```python
from build123d import *

# Parameters (mm, degrees)
BOSS_EXTRUDE1_DEPTH            = 3
SKETCH3_R                      = 4
CUT_EXTRUDE1_DEPTH             = 3
CBORE_FOR_M2_SHCS1_D           = 2.4
CBORE_FOR_M2_SHCS1_DEPTH       = 3
CBORE_FOR_M2_SHCS1_CBORE_D     = 4.4
CBORE_FOR_M2_SHCS1_CBORE_DEPTH = 2
CBORE_FOR_M2_SHCS1_TIP         = 0.721032743
CUT_EXTRUDE2_DEPTH             = 3
SKETCH7_W                      = 6
SKETCH7_H                      = 10
CUT_EXTRUDE3_DEPTH             = 3
CUT_EXTRUDE4_DEPTH             = 3
CBORE_FOR_M2_SHCS2_D           = 2.4
CBORE_FOR_M2_SHCS2_DEPTH       = 3
CBORE_FOR_M2_SHCS2_CBORE_D     = 4.4
CBORE_FOR_M2_SHCS2_CBORE_DEPTH = 2
CBORE_FOR_M2_SHCS2_TIP         = 0.721032743
SALIENTE_EXTRUIR2_DEPTH        = 3
CORTAR_EXTRUIR2_DEPTH          = 25
CORTAR_EXTRUIR3_DEPTH          = 8
CORTAR_EXTRUIR3_DEPTH_BACK     = 1
SALIENTE_EXTRUIR3_DEPTH        = 3
CORTAR_EXTRUIR4_DEPTH          = 32
CORTAR_EXTRUIR4_DEPTH_BACK     = 3
CORTAR_EXTRUIR5_DEPTH          = 33
CORTAR_EXTRUIR5_DEPTH_BACK     = 16
CORTAR_EXTRUIR6_DEPTH          = 36
CORTAR_EXTRUIR6_DEPTH_BACK     = 57
CROQUIS10_W                    = 8
CROQUIS10_H                    = 20.24327749
CROQUIS11_W                    = 22.516217108
CROQUIS11_H                    = 6.585791746
SALIENTE_EXTRUIR4_DEPTH        = 3
CORTAR_EXTRUIR7_DEPTH          = 12
CORTAR_EXTRUIR7_DEPTH_BACK     = 26
CORTAR_EXTRUIR8_DEPTH          = 37
CORTAR_EXTRUIR8_DEPTH_BACK     = 23
CORTAR_EXTRUIR10_DEPTH         = 10
CORTAR_EXTRUIR10_DEPTH_BACK    = 13
CROQUIS14_W                    = 22.056135014
CROQUIS14_H                    = 3.895510455
CORTAR_EXTRUIR11_DEPTH         = 15
CORTAR_EXTRUIR11_DEPTH_BACK    = 12
CROQUIS15_W                    = 4.816352665
CROQUIS15_H                    = 5.664480242
CORTAR_EXTRUIR12_DEPTH         = 33
CORTAR_EXTRUIR12_DEPTH_BACK    = 21
CORTAR_EXTRUIR18_DEPTH         = 52
CORTAR_EXTRUIR18_DEPTH_BACK    = 75
CORTAR_EXTRUIR19_DEPTH         = 24
CORTAR_EXTRUIR19_DEPTH_BACK    = 67
CORTAR_EXTRUIR20_DEPTH         = 39
CORTAR_EXTRUIR20_DEPTH_BACK    = 62
SALIENTE_EXTRUIR7_DEPTH        = 3
SALIENTE_EXTRUIR9_DEPTH        = 3
SALIENTE_EXTRUIR10_DEPTH       = 3


with BuildPart() as part:
    # Sketch2 → Boss-Extrude1 (new body)
    with BuildSketch(Plane.XY):
        Polygon((-5.811176978, -98.599598559), (-3.564526654, -100.58433119), (7.435473346, -100.58433119), (9.68212367, -98.599598559), (21.318847535, -4.961831578), (21.935473346, 5), (21.935473346, 45), (21.193771081, 54.944681764), (15.17717561, 95.055318236), (9.435473346, 100), (-5.564526654, 100), (-11.306228919, 95.055318236), (-17.32282439, 54.944681764), (-18.064526654, 45), (-18.064526654, 5), (-17.447900844, -4.961831578), align=None)
    extrude(amount=BOSS_EXTRUDE1_DEPTH)

    # Sketch3 → Cut-Extrude1 (cut)
    with BuildSketch(Plane.XY.offset(3)):
        with Locations((1.935473346, 25)):
            Circle(SKETCH3_R)
    extrude(amount=-CUT_EXTRUDE1_DEPTH, mode=Mode.SUBTRACT)

    # CBORE for M2 SHCS1
    with Locations(Plane.XY.offset(3)):
        with Locations((1.935473346, 33), (9.935473346, 25), (1.935473346, 17), (-6.064526654, 25)):
            CounterBoreHole(CBORE_FOR_M2_SHCS1_D / 2, CBORE_FOR_M2_SHCS1_CBORE_D / 2, CBORE_FOR_M2_SHCS1_CBORE_DEPTH, depth=CBORE_FOR_M2_SHCS1_DEPTH)
            with Locations((0, 0, -(CBORE_FOR_M2_SHCS1_DEPTH + CBORE_FOR_M2_SHCS1_TIP / 2))):  # 118° drill point
                Cone(0, CBORE_FOR_M2_SHCS1_D / 2, CBORE_FOR_M2_SHCS1_TIP, mode=Mode.SUBTRACT)

    # Sketch6 → Cut-Extrude2 (cut)
    with BuildSketch(Plane.XY.offset(3)):
        Polygon((-10.32282439, 54.944681764), (-2.592495206, 54.944681764), (-0.592495206, 56.944681764), (-0.592495206, 77.986977382), (-2.570367912, 80.283658288), (-6.413140682, 80.860074204), (-8.687694294, 79.178882404), (-12.026143484, 56.92255447), align=None)
        Polygon((15.841153071, 56.92255447), (12.502703881, 79.178882404), (10.22815027, 80.860074204), (6.385377499, 80.283658288), (4.407504794, 77.986977382), (4.407504794, 56.944681764), (6.407504794, 54.944681764), (14.137833977, 54.944681764), align=None)
        Polygon((-4.417484259, 94.313615971), (8.232493846, 94.313615971), (10.529174752, 92.335743265), (11.167639805, 88.07930958), (9.486448005, 85.804755968), (1.907504794, 84.667914487), (-5.671438417, 85.804755968), (-7.352630217, 88.07930958), (-6.714165164, 92.335743265), align=None)
    extrude(amount=-CUT_EXTRUDE2_DEPTH, mode=Mode.SUBTRACT)

    # Sketch7 → Cut-Extrude3 (cut)
    with BuildSketch(Plane.XY.offset(3)):
        with Locations((1.935473346, -85.58433119)):
            Rectangle(SKETCH7_W, SKETCH7_H)
    extrude(amount=-CUT_EXTRUDE3_DEPTH, mode=Mode.SUBTRACT)

    # Sketch8 → Cut-Extrude4 (cut)
    with BuildSketch(Plane.XY.offset(3)):
        Polygon((-8.447900844, -4.961831578), (12.318847535, -4.961831578), (1.935473346, -24.483157151), align=None)
        Polygon((15.880690917, -8.470858754), (8.202586605, -69.961831578), (4.435473346, -69.961831578), (4.435473346, -29.183297302), align=None)
        Polygon((-12.009744226, -8.470858754), (-4.331639914, -69.961831578), (-0.564526654, -69.961831578), (-0.564526654, -29.183297302), align=None)
    extrude(amount=-CUT_EXTRUDE4_DEPTH, mode=Mode.SUBTRACT)

    # CBORE for M2 SHCS2
    with Locations(Plane.XY.offset(3)):
        with Locations((-3.715014103, -74.923663156), (7.581217459, -74.961831578), (-11.190875883, -5.696432584), (15.095204577, -5.939721308), (1.907504794, 81.167914487)):
            CounterBoreHole(CBORE_FOR_M2_SHCS2_D / 2, CBORE_FOR_M2_SHCS2_CBORE_D / 2, CBORE_FOR_M2_SHCS2_CBORE_DEPTH, depth=CBORE_FOR_M2_SHCS2_DEPTH)
            with Locations((0, 0, -(CBORE_FOR_M2_SHCS2_DEPTH + CBORE_FOR_M2_SHCS2_TIP / 2))):  # 118° drill point
                Cone(0, CBORE_FOR_M2_SHCS2_D / 2, CBORE_FOR_M2_SHCS2_TIP, mode=Mode.SUBTRACT)

    # Croquis2 → Saliente-Extruir2 (add)
    with BuildSketch(Plane.XY):
        Polygon((18.794620774, 54.944681764), (-14.944396603, 54.944681764), (-7.478946257, 96.267482636), (12.143583194, 96.267482636), align=None)
    extrude(amount=SALIENTE_EXTRUIR2_DEPTH)

    # Croquis3 → Cortar-Extruir2 (cut)
    with BuildSketch(Plane.XY):
        Polygon((3.935473346, 75), (15.193771081, 54.944681764), (9.17717561, 95.055318236), (3.935473346, 95.055318236), align=None)
        Polygon((-5.306228919, 95.055318236), (-11.32282439, 54.944681764), (-0.064526654, 75), (-0.064526654, 95.055318236), align=None)
        Polygon((1.935473346, 67.392726007), (10.193771081, 54.944681764), (-6.32282439, 54.944681764), align=None)
    extrude(amount=CORTAR_EXTRUIR2_DEPTH, mode=Mode.SUBTRACT)

    # Croquis4 → Cortar-Extruir3 (cut, two sides: drawn at the far end of the back side and taken through both)
    with BuildSketch(Plane.XY.offset(-CORTAR_EXTRUIR3_DEPTH_BACK)):
        Polygon((-16.681169013, 74.945942972), (0, 74.945942972), (20.337076697, 74.945942972), (20.337076697, 106.026068233), (-16.681169013, 106.026068233), align=None)
    extrude(amount=CORTAR_EXTRUIR3_DEPTH + CORTAR_EXTRUIR3_DEPTH_BACK, mode=Mode.SUBTRACT)

    # Croquis5 → Saliente-Extruir3 (add)
    with BuildSketch(Plane.XY):
        Polygon((-14.322635208, 74.945942972), (18.1935819, 74.945942972), (18.1935819, 53.950721804), (-16.161111671, 53.950721804), align=None)
    extrude(amount=SALIENTE_EXTRUIR3_DEPTH)

    # Croquis8 → Cortar-Extruir4 (cut, two sides: drawn at the far end of the back side and taken through both)
    with BuildSketch(Plane.XY.offset(-CORTAR_EXTRUIR4_DEPTH_BACK)):
        Polygon((-14.322635208, 74.945942972), (-15.372635208, 67.945942972), (-9.322635208, 74.945942972), align=None)
        Polygon((18.1935819, 74.945942972), (13.1935819, 74.945942972), (19.2435819, 67.945942972), align=None)
    extrude(amount=CORTAR_EXTRUIR4_DEPTH + CORTAR_EXTRUIR4_DEPTH_BACK, mode=Mode.SUBTRACT)

    # Croquis9 → Cortar-Extruir5 (cut, two sides: drawn at the far end of the back side and taken through both)
    with BuildSketch(Plane.XY.offset(-CORTAR_EXTRUIR5_DEPTH_BACK)):
        Polygon((-9.322635208, 67.945942972), (-9.322635208, 70.912384295), (13.1935819, 70.912384295), (13.1935819, 67.945942972), (13.1935819, 64.326592549), (-9.322635208, 64.326592549), align=None)
    extrude(amount=CORTAR_EXTRUIR5_DEPTH + CORTAR_EXTRUIR5_DEPTH_BACK, mode=Mode.SUBTRACT)

    # Croquis10 → Cortar-Extruir6 (cut, two sides: drawn at the far end of the back side and taken through both)
    with BuildSketch(Plane.XY.offset(-CORTAR_EXTRUIR6_DEPTH_BACK)):
        with Locations((-5.322635208, 49.537038019)):
            Rectangle(CROQUIS10_W, CROQUIS10_H)
        with Locations((9.1935819, 49.537038019)):
            Rectangle(CROQUIS10_W, CROQUIS10_H)
    extrude(amount=CORTAR_EXTRUIR6_DEPTH + CORTAR_EXTRUIR6_DEPTH_BACK, mode=Mode.SUBTRACT)

    # Croquis11 → Saliente-Extruir4 (add)
    with BuildSketch(Plane.XY):
        with Locations((1.935473346, 67.619488422)):
            Rectangle(CROQUIS11_W, CROQUIS11_H)
    extrude(amount=SALIENTE_EXTRUIR4_DEPTH)

    # Croquis12 → Cortar-Extruir7 (cut, two sides: drawn at the far end of the back side and taken through both)
    with BuildSketch(Plane.XY.offset(-CORTAR_EXTRUIR7_DEPTH_BACK)):
        Polygon((-15.372635208, 67.945942972), (-9.322635208, 74.945942972), (-5.822635208, 74.945942972), (-17.32282439, 54.944681764), align=None)
    extrude(amount=CORTAR_EXTRUIR7_DEPTH + CORTAR_EXTRUIR7_DEPTH_BACK, mode=Mode.SUBTRACT)

    # Croquis13 → Cortar-Extruir8 (cut, two sides: drawn at the far end of the back side and taken through both)
    with BuildSketch(Plane.XY.offset(-CORTAR_EXTRUIR8_DEPTH_BACK)):
        Polygon((13.1935819, 74.945942972), (9.6935819, 74.945942972), (21.193771081, 54.944681764), (19.2435819, 67.945942972), align=None)
    extrude(amount=CORTAR_EXTRUIR8_DEPTH + CORTAR_EXTRUIR8_DEPTH_BACK, mode=Mode.SUBTRACT)

    # Croquis14 → Cortar-Extruir10 (cut, two sides: drawn at the far end of the back side and taken through both)
    with BuildSketch(Plane.XY.offset(-CORTAR_EXTRUIR10_DEPTH_BACK)):
        with Locations((5.205432299, 72.998187745)):
            Rectangle(CROQUIS14_W, CROQUIS14_H)
    extrude(amount=CORTAR_EXTRUIR10_DEPTH + CORTAR_EXTRUIR10_DEPTH_BACK, mode=Mode.SUBTRACT)

    # Croquis15 → Cortar-Extruir11 (cut, two sides: drawn at the far end of the back side and taken through both)
    with BuildSketch(Plane.XY.offset(-CORTAR_EXTRUIR11_DEPTH_BACK)):
        with Locations((-8.230811541, 73.882672638)):
            Rectangle(CROQUIS15_W, CROQUIS15_H)
    extrude(amount=CORTAR_EXTRUIR11_DEPTH + CORTAR_EXTRUIR11_DEPTH_BACK, mode=Mode.SUBTRACT)

    # Croquis16 → Cortar-Extruir12 (cut, two sides: drawn at the far end of the back side and taken through both)
    with BuildSketch(Plane.XY.offset(-CORTAR_EXTRUIR12_DEPTH_BACK)):
        Polygon((-8.062449324, 71.050432517), (-7.062449324, 71.050432517), (-17.32282439, 54.944681764), align=None)
        Polygon((11.933396016, 71.050432517), (10.933396016, 71.050432517), (21.193771081, 54.944681764), align=None)
    extrude(amount=CORTAR_EXTRUIR12_DEPTH + CORTAR_EXTRUIR12_DEPTH_BACK, mode=Mode.SUBTRACT)

    # Croquis18 → Cortar-Extruir18 (cut, two sides: drawn at the far end of the back side and taken through both)
    with BuildSketch(Plane.XY.offset(-CORTAR_EXTRUIR18_DEPTH_BACK)):
        Polygon((-7.062449324, 71.050432517), (-5.062449324, 71.050432517), (-7.826924714, 69.850432517), align=None)
        Polygon((10.933396016, 71.050432517), (8.933396016, 71.050432517), (11.697871405, 69.850432517), align=None)
    extrude(amount=CORTAR_EXTRUIR18_DEPTH + CORTAR_EXTRUIR18_DEPTH_BACK, mode=Mode.SUBTRACT)

    # Croquis20 → Cortar-Extruir19 (cut, two sides: drawn at the far end of the back side and taken through both)
    with BuildSketch(Plane.XY.offset(-CORTAR_EXTRUIR19_DEPTH_BACK)):
        Polygon((21.193771081, 54.944681764), (20.226639816, 56.462791483), (21.564622213, 49.972340882), align=None)
        Polygon((-17.32282439, 54.944681764), (-16.355693125, 56.462791483), (-17.693675522, 49.972340882), align=None)
    extrude(amount=CORTAR_EXTRUIR19_DEPTH + CORTAR_EXTRUIR19_DEPTH_BACK, mode=Mode.SUBTRACT)

    # Croquis21 → Cortar-Extruir20 (cut, two sides: drawn at the far end of the back side and taken through both)
    with BuildSketch(Plane.XY.offset(-CORTAR_EXTRUIR20_DEPTH_BACK)):
        Polygon((-9.322635208, 39.415399274), (-12.822635208, 39.415399274), (-9.322635208, 59.658676764), align=None)
        Polygon((13.1935819, 39.415399274), (16.6935819, 39.415399274), (13.1935819, 59.658676764), align=None)
    extrude(amount=CORTAR_EXTRUIR20_DEPTH + CORTAR_EXTRUIR20_DEPTH_BACK, mode=Mode.SUBTRACT)

    # Croquis23 → Saliente-Extruir7 (add)
    with BuildSketch(Plane.XY):
        Polygon((-9.322635208, 59.658676764), (-9.581980564, 58.158676764), (-7.822635208, 59.658676764), align=None)
        Polygon((13.1935819, 59.658676764), (11.6935819, 59.658676764), (13.452927256, 58.158676764), align=None)
    extrude(amount=SALIENTE_EXTRUIR7_DEPTH)

    # Croquis24 → Saliente-Extruir9 (add)
    with BuildSketch(Plane.XY):
        Polygon((-12.822635208, 39.415399274), (-11.022635208, 39.415399274), (-12.476841401, 41.415399274), align=None)
        Polygon((-1.322635208, 39.415399274), (-1.322635208, 40.415399274), (-2.322635208, 39.415399274), align=None)
        Polygon((5.1935819, 39.415399274), (6.1935819, 39.415399274), (5.1935819, 40.415399274), align=None)
        Polygon((14.8935819, 39.415399274), (16.347788092, 41.415399274), (16.6935819, 39.415399274), align=None)
    extrude(amount=SALIENTE_EXTRUIR9_DEPTH)

    # Croquis25 → Saliente-Extruir10 (add)
    with BuildSketch(Plane.XY):
        Polygon((5.1935819, 59.658676764), (5.1935819, 58.658676764), (7.1935819, 59.658676764), align=None)
        Polygon((-1.322635208, 58.658676764), (-3.322635208, 59.658676764), (-1.322635208, 59.658676764), align=None)
    extrude(amount=SALIENTE_EXTRUIR10_DEPTH)


solid = part.part
```
Geometry: final body of the model. Coordinates: model frame, mm. A direction names the side the tool comes from. Give positions to 0.01 mm unless a question says otherwise; leave off trailing zeros. Loops run counter-clockwise (first coordinate to the right, second up) from the corner with the lowest first, then second, coordinate; pieces in that order, holes last. Notation, with made-up numbers: (59, 88) - (89, 88) arc R25 cw to (89, 119) - close; hole circle Ø11 at (-16, 8.25). An arc over 180 degrees is marked (long way). Answer as CSV lines item,"result". Start each with the question number.
(1) Section query C-C (z = 1.8). Give the number of separate pieces and of enclosed holes in the cut face, and give its area (3 significant figures).
(2) Mould query, pull axis Y, two halves, no side actions, for faces 1 (the face through (21.935, 25, 1)), 2 (the face through (2, -80.584, 2)), 3 (the face through (2, -100.584, 1)). Classes: +Y half, -Y half, draft (parallel to the pull), parting line (faces both ways), or undercut.
(3) Section query B-B (y = -12.5). Output: boundary loops of the cut face in (x, z), and give its area (3 significant figures).
(4) Pin query (flat end, axial travel): P1, Ø10, axis at x = -3.5, y = -71, coming from the -Z side; P2, Ø3, axis at x = -3.72, y = -74.92, coming from the +Z side; P3, Ø0.9, axis at x = 11, z = 1, coming from the +Y side. Return the tip coordinate at first contact, or that it passes through.
(5) Reachability of faces 4 (the face through (5.194, 49, 1)), 5 (the face through (-5, 24, 1)), 6 (the face through (-18.065, 25, 1)) from +Z, -Z, +X, -X, +Y, -Y: full face, straight path, thin tool, end or side. Return the list, or none.
(6) Ray query, line 1 along X through (y, z) = (-62.5, 0.65); line 2 along X through (y, z) = (-33.5, 0.15); line 3 along X through (y, z) = (-7.5, 1.45). Return the intervals inside material, ascending. Write a range as [from, to].
(7) Section query A-A (y = -87). Output: boundary loops of the cut face in (x, z).
Worked answers:
1,separate pieces,"1"
1,enclosed holes,"15"
1,area,"3,880 mm^2"
2,face 1,"draft"
2,face 2,"undercut"
2,face 3,"-Y half"
3,outline,"(-16.51, 0) - (-11.51, 0) - (-11.51, 3) - (-16.51, 3) - close; (-9.78, 0) - (-4.44, 0) - (-4.44, 3) - (-9.78, 3) - close; (8.31, 0) - (13.65, 0) - (13.65, 3) - (8.31, 3) - close; (15.38, 0) - (20.38, 0) - (20.38, 3) - (15.38, 3) - close"
3,area,"62.1 mm^2"
4,P1,"stops at z = 0"
4,P2,"stops at z = 1"
4,P3,"stops at y = 70.35"
5,face 4,"+Z, -Z"
5,face 5,"+Z"
5,face 6,"+Z, -Z, -X, +Y, -Y"
6,line 1,"x = [-10.3, -5.26], [-0.56, 4.44], [9.13, 14.17]"
6,line 2,"x = [-13.9, -8.88], [-0.56, 4.44], [12.76, 17.77]"
6,line 3,"x = [-17.13, -12.45], [-9.93, -7.1], [10.97, 13.54], [16.65, 21]"
7,outline,"(-7.25, 0) - (-1.06, 0) - (-1.06, 3) - (-7.25, 3) - close; (4.94, 0) - (11.12, 0) - (11.12, 3) - (4.94, 3) - close"
